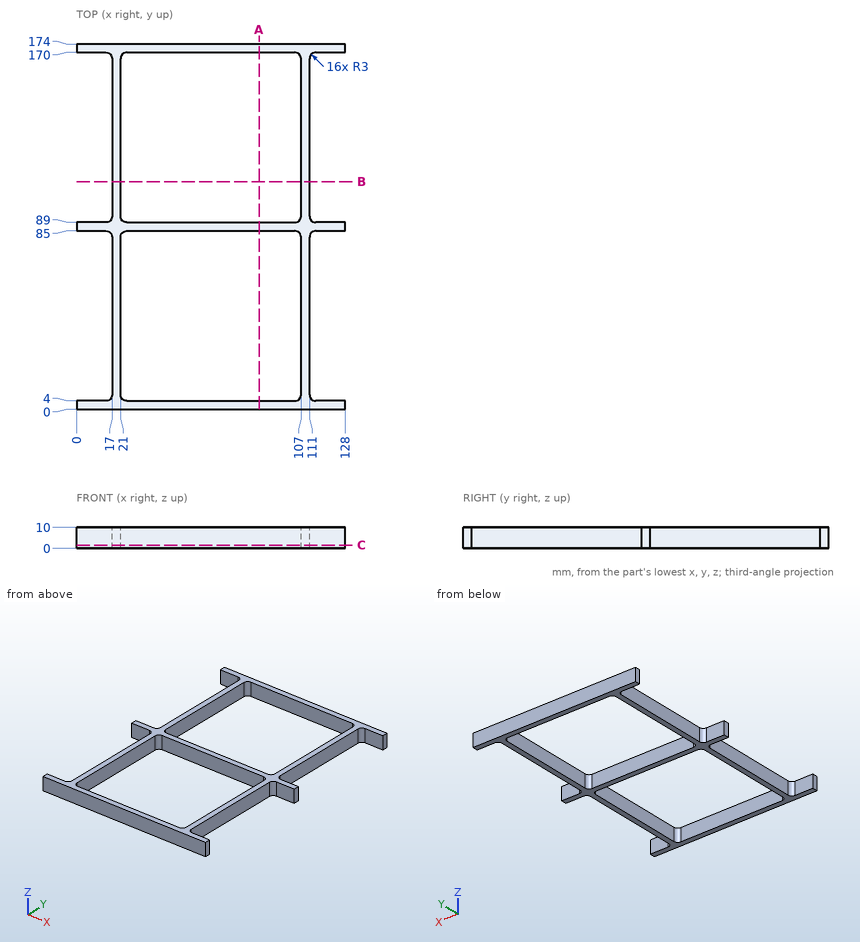
Here's the drawing with two shaded views (mm, measured from the low corner). I have some questions. Give positions to 0.01 mm unless a question says otherwise; leave off trailing zeros. Write each loop counter-clockwise with the first axis right and the second up, starting at its lowest first coordinate (ties: lowest second). Pieces come first, ordered by that corner, then holes. Notation, with made-up numbers: (29.25, 58.25) -> (49.25, 58.25) arc R35 cw to (49.25, 90.25) -> close; hole circle Ø2 at (35, 67.25). An arc over 180 degrees is marked (long way). Use one line per item in the form item = value.
1) Suppose I cut it at B-B (y = 108.5). Please give me the cut outline in (x, z).
Verdict:
outline = (17, 0) -> (21, 0) -> (21, 10) -> (17, 10) -> close; (107, 0) -> (111, 0) -> (111, 10) -> (107, 10) -> close
2) Suppose I cut it at A-A (x = 87). Please give me the cut outline in (y, z), and give its area (3 significant figures).
Verdict:
outline = (0, 0) -> (4, 0) -> (4, 10) -> (0, 10) -> close; (85, 0) -> (89, 0) -> (89, 10) -> (85, 10) -> close; (170, 0) -> (174, 0) -> (174, 10) -> (170, 10) -> close
area = 120 mm2
3) Suppose I cut it at C-C (z = 1.5). Give the number of separate pieces and of enclosed holes in the cut face, and give its area (3 significant figures).
Verdict:
separate_pieces = 1
enclosed_holes = 2
area = 2,860 mm2
4) If I drill on L1, parallel to Y at x = 71.5, z = 8; L2, parallel to X at y = 56, z = 2, over which ranges is the centre line in solid material (lowest first)? Write a range as [from, to].
Verdict:
L1 = [0, 4], [85, 89], [170, 174]
L2 = [17, 21], [107, 111]
5) I'm going to push flat-ended pins straight in: pin 1 (1 mm diameter, centred on y = 105, z = 2.5, fed in from +X); pin 2 (5 mm diameter, centred on y = 111, z = 3, fed in from -X); pin 3 (3 mm diameter, centred on x = 118.5, z = 3, fed in from -Y). Where does each tip first touch, or does it pass through?
Verdict:
pin_1 = 111
pin_2 = 17
pin_3 = 0
